from build123d import *


with BuildPart() as part:
    # Sketch1 → Revolve1 (revolve)
    with BuildSketch(Plane.XY, mode=Mode.PRIVATE) as revolve1_sk:
        Polygon((12.5, 73.991760417), (0, 73.991760417), (0, -126.008239583), (12.5, -126.008239583), (12.5, -76.008239583), (16, -76.008239583), (16, 23.991760417), (12.5, 23.991760417), align=None)
        with BuildLine():
            Line((0, 86.491760417), (0, 73.991760417))
            Line((0, 73.991760417), (12.5, 73.991760417))
            ThreePointArc((12.5, 73.991760417), (8.838834765, 82.830595182), (0, 86.491760417))
        make_face()
        with BuildLine():
            Line((12.5, -126.008239583), (0, -126.008239583))
            Line((0, -126.008239583), (0, -138.508239583))
            ThreePointArc((0, -138.508239583), (8.838834765, -134.847074348), (12.5, -126.008239583))
        make_face()
    revolve(revolve1_sk.sketch.rotate(Axis((0, 86.491760417, 0), (0, -1, 0)), 90), axis=Axis((0, 86.491760417, 0), (0, -1, 0)))


solid = part.part
Geometry check sheet. Reference: the model listing, model coordinates, mm. A direction names the side the tool comes from. Give positions to 0.01 mm unless a question says otherwise; leave off trailing zeros. Write each loop counter-clockwise with the first axis right and the second up, starting at its lowest first coordinate (ties: lowest second). Pieces come first, ordered by that corner, then holes. Notation, with made-up numbers: M -34.5,-5.75 L 10.5,-5.75 A12 cw 10.5,17.25 Z; hole C 20,-3 d2. An arc over 180 degrees is marked long. One line per question, with ' | ' between items.
1. Scan lines: line 1 along Y through (x, z) = (-13.5, 7); line 2 along Z through (x, y) = (1, 56.5); line 3 along Z through (x, y) = (0.5, -64). Record each from-to range of solid material in increasing order. Write a range as from..to.
Ans:
line 1: -76.01..23.99 | line 2: -12.46..12.46 | line 3: -15.99..15.99
2. Mould release check, pull along X, two halves, no side actions. Record for faces 4 (the face through (-3.755, -100.658, 11.923)), 5 (the face through (8, 23.992, -10)): released by +X, released by -X, zero draft, split by the parting line, or undercut.
Ans:
face 4: split by the parting line | face 5: zero draft
3. Cross-section at A-A (x = 0). Enter the section's corners in (y, z), plus the area to 3 significant figures.
Ans:
outline: M -126.01,-12.5 L -76.01,-12.5 L -76.01,-16 L 23.99,-16 L 23.99,-12.5 L 73.99,-12.5 A12.5 ccw 73.99,12.5 L 23.99,12.5 L 23.99,16 L -76.01,16 L -76.01,12.5 L -126.01,12.5 A12.5 ccw Z | area: 6,190 mm2
4. Gauge pin test, flat ends, axial feed: pin 1 (6 mm diameter, centred on x = 10.5, y = -22, fed in from -Z); pin 2 (10 mm diameter, centred on x = 9.5, z = 11.5, fed in from +Y); pin 3 (2 mm diameter, centred on y = 2.5, z = -4.5, fed in from -X). Record the tip position at first contact, or that the pin passes through.
Ans:
pin 1: z = -14.13 | pin 2: y = 81.6 | pin 3: x = -15.61
5. Set-up check for faces 1 (the face through (-3.755, 49.342, 11.923)), 2 (the face through (15.62, -25.31, -3.47)), 3 (the face through (8, -76.008, 10)): record each of +Z, -Z, +X, -X, +Y, -Y from which the full face is reachable in a straight line by a thin tool's end or side.
Ans:
face 1: +Y | face 2: +Y, -Y | face 3: -Y
6. Cross-section at D-D (z = 9.5). Enter the section's corners in (x, y).
Ans:
outline: M -12.87,-76.01 L -8.12,-76.01 L -8.12,-126.01 A8.12 ccw 8.12,-126.01 L 8.12,-76.01 L 12.87,-76.01 L 12.87,23.99 L 8.12,23.99 L 8.12,73.99 A8.12 ccw -8.12,73.99 L -8.12,23.99 L -12.87,23.99 Z
7. Cross-section at B-B (z = 0). Enter the section's corners in (x, y), plus the area to 3 significant figures.
Ans:
outline: M -16,-76.01 L -12.5,-76.01 L -12.5,-126.01 A12.5 ccw 12.5,-126.01 L 12.5,-76.01 L 16,-76.01 L 16,23.99 L 12.5,23.99 L 12.5,73.99 A12.5 ccw -12.5,73.99 L -12.5,23.99 L -16,23.99 Z | area: 6,190 mm2
8. Cross-section at C-C (y = 44). Enter the section's corners in (x, z), plus the area to 3 significant figures.
Ans:
outline: C 0,0 d25 | area: 491 mm2
